For this review, take the finished solid that the model builds, in its own axes (mm). A direction names the side the tool comes from. Coordinates: 2 decimals unless noted, no trailing zeros. Write each loop counter-clockwise with the first axis right and the second up, starting at its lowest first coordinate (ties: lowest second). Pieces come first, ordered by that corner, then holes. Notation, with made-up numbers: (20, 15) - (75, 15) arc R28 cw to (75, 47) - close; hole circle Ø10 at (53.5, 50.5). An arc over 180 degrees is marked (long way). Write each question's results on one line, items separated by ' | '.
from build123d import *

# Parameters (mm, degrees)
CUT_EXTRUDE3_DEPTH           = 60
CUT_EXTRUDE5_DEPTH           = 2
CUT_EXTRUDE5_DEPTH_BACK      = 30
SKETCH9_R                    = 38
SKETCH9_R_2                  = 23
SKETCH19_W                   = 12
SKETCH19_H                   = 36.5
CUT_REVOLVE2_ANGLE           = 65
CUT_REVOLVE2_OTHER_WAY_ANGLE = 65
SKETCH21_W                   = 3.25
SKETCH21_H                   = 4
BOSS_EXTRUDE3_DEPTH          = 1.35
CIRPATTERN1_COUNT            = 5
CUT_EXTRUDE9_START           = -5
CUT_EXTRUDE9_DEPTH           = 5
SKETCH23_R                   = 10.5
CUT_EXTRUDE10_DEPTH          = 10
SKETCH24_W                   = 15
SKETCH24_H                   = 8
BOSS_EXTRUDE4_DEPTH          = 8
SKETCH26_W                   = 10
SKETCH26_H                   = 6
CUT_EXTRUDE11_DEPTH          = 10
SKETCH27_W                   = 4
SKETCH27_H                   = 5
CUT_EXTRUDE12_DEPTH          = 5
CUT_EXTRUDE14_DEPTH          = 2
CUT_EXTRUDE14_DEPTH_BACK     = 30
SKETCH29_R                   = 1
CUT_EXTRUDE15_DEPTH          = 15
FILLET1_R                    = 6
FILLET2_R                    = 8


# Read off the part's stored shape, not the designer's step: Cut-Extrude9
with BuildPart() as part:
    # Sketch1 → Revolve1 (revolve)
    with BuildSketch(Plane.XY, mode=Mode.PRIVATE) as revolve1_sk:
        with BuildLine():
            Line((0, 63.427876097), (32, 63.427876097))
            ThreePointArc((32, 63.427876097), (37.656854249, 61.084730346), (40, 55.427876097))
            Line((40, 55.427876097), (40, 28.846818009))
            ThreePointArc((40, 28.846818009), (38.792081772, 24.082439968), (35.460140376, 20.469057744))
            Line((35.460140376, 20.469057744), (28.539859624, 15.958818353))
            ThreePointArc((28.539859624, 15.958818353), (25.207918228, 12.345436129), (24, 7.581058088))
            Line((24, 7.581058088), (24, 3.25))
            Line((24, 3.25), (24.35, 3))
            Line((24.35, 3), (24.35, 0))
            Line((24.35, 0), (22.5, 0))
            Line((22.5, 0), (22.5, 12.5))
            ThreePointArc((22.5, 12.5), (22.353553391, 12.853553391), (22, 13))
            Line((22, 13), (0, 13))
            Line((0, 13), (0, 63.427876097))
        make_face()
    revolve(revolve1_sk.sketch.rotate(Axis((0, 0, 0), (0, 1, 0)), 90), axis=Axis((0, 0, 0), (0, 1, 0)))

    # Sketch11 → Cut-Extrude3 (cut)
    with BuildSketch(Plane(origin=(0, 13, 0), x_dir=(-1, 0, 0), z_dir=(0, -1, 0))):
        with BuildLine():
            Line((-21, 0), (21, 0))
            ThreePointArc((21, 0), (0, 21), (-21, 0))
        make_face()
    extrude(amount=-CUT_EXTRUDE3_DEPTH, mode=Mode.SUBTRACT)

    # Sketch9 → Cut-Extrude5 (cut, two sides: drawn at the far end of the back side and taken through both)
    with BuildSketch(Plane(origin=(0, 55.427876097, 0), x_dir=(1, 0, 0), z_dir=(0, 1, 0)).offset(-CUT_EXTRUDE5_DEPTH_BACK)):
        with Locations(Location((0, 0, 0), (0, 0, 270))):
            Circle(SKETCH9_R)
        with Locations(Location((0, 0, 0), (0, 0, 270))):
            Circle(SKETCH9_R_2, mode=Mode.SUBTRACT)
    extrude(amount=CUT_EXTRUDE5_DEPTH + CUT_EXTRUDE5_DEPTH_BACK, mode=Mode.SUBTRACT)

    # Sketch19 → Cut-Revolve2 (revolve, cut)
    with BuildSketch(Plane(origin=(0, 0, 0), x_dir=(0, 0, -1), z_dir=(1, 0, 0))):
        with Locations((-41.064715832, 37.177876097)):
            Rectangle(SKETCH19_W, SKETCH19_H)
    revolve(axis=Axis((0, 0, 0), (0, 1, 0)), revolution_arc=CUT_REVOLVE2_ANGLE, mode=Mode.SUBTRACT)

    # Sketch19 → Cut-Revolve2 other way (revolve, cut)
    with BuildSketch(Plane(origin=(0, 0, 0), x_dir=(0, 0, -1), z_dir=(1, 0, 0))):
        with Locations((-41.064715832, 37.177876097)):
            Rectangle(SKETCH19_W, SKETCH19_H)
    revolve(axis=Axis((0, 0, 0), (0, -1, 0)), revolution_arc=CUT_REVOLVE2_OTHER_WAY_ANGLE, mode=Mode.SUBTRACT)

    # Sketch21 → Boss-Extrude3 (add)
    with BuildSketch(Plane(origin=(0, 0, 22.5), x_dir=(-1, 0, 0), z_dir=(0, 0, -1))):
        with Locations((0, 2)):
            Rectangle(SKETCH21_W, SKETCH21_H)
    boss_extrude3 = extrude(amount=BOSS_EXTRUDE3_DEPTH)

    # CirPattern1: Boss-Extrude3 ×5 about axis
    cirpattern1_axis = Axis((0, 0, 0), (0, 1, 0))
    for i in range(1, CIRPATTERN1_COUNT):
        add(boss_extrude3.rotate(cirpattern1_axis, i * 360 / CIRPATTERN1_COUNT))

    # Cut-Extrude9 outline → Cut-Extrude9 (cut)
    with BuildSketch(Plane(origin=(0, 63.427876097, 0), x_dir=(1, 0, 0), z_dir=(0, 1, 0)).offset(CUT_EXTRUDE9_START)):
        with BuildLine():
            ThreePointArc((40, 0), (0, 40), (-40, 0))
            Line((-40, 0), (-21, 0))
            ThreePointArc((-21, 0), (0, 21), (21, 0))
            Line((21, 0), (40, 0))
        make_face()
    extrude(amount=CUT_EXTRUDE9_DEPTH, mode=Mode.SUBTRACT)

    # Sketch23 → Cut-Extrude10 (cut)
    with BuildSketch(Plane(origin=(0, 0, -40), x_dir=(-1, 0, 0), z_dir=(0, 0, -1))):
        with Locations((0, 42.137876097)):
            Circle(SKETCH23_R)
    extrude(amount=-CUT_EXTRUDE10_DEPTH, mode=Mode.SUBTRACT)

    # Sketch24 → Boss-Extrude4 (add)
    with BuildSketch(Plane(origin=(0, 58.427876097, 0), x_dir=(1, 0, 0), z_dir=(0, 1, 0))):
        with Locations((0, 30)):
            Rectangle(SKETCH24_W, SKETCH24_H)
    extrude(amount=-BOSS_EXTRUDE4_DEPTH)

    # Sketch26 → Cut-Extrude11 (cut)
    with BuildSketch(Plane(origin=(0, 58.427876097, 0), x_dir=(1, 0, 0), z_dir=(0, 1, 0))):
        with Locations((0, 30)):
            Rectangle(SKETCH26_W, SKETCH26_H)
    extrude(amount=-CUT_EXTRUDE11_DEPTH, mode=Mode.SUBTRACT)

    # Sketch27 → Cut-Extrude12 (cut)
    with BuildSketch(Plane(origin=(7.5, 0, 0), x_dir=(0, 0, -1), z_dir=(1, 0, 0))):
        with Locations((30, 53.927876097)):
            Rectangle(SKETCH27_W, SKETCH27_H)
    extrude(amount=-CUT_EXTRUDE12_DEPTH, mode=Mode.SUBTRACT)

    # Sketch28 → Cut-Extrude14 (cut, two sides: drawn at the far end of the back side and taken through both)
    with BuildSketch(Plane(origin=(0, 55.427876097, 0), x_dir=(1, 0, 0), z_dir=(0, 1, 0)).offset(-CUT_EXTRUDE14_DEPTH_BACK)):
        with BuildLine():
            Line((-22.912878475, -2), (22.912878475, -2))
            ThreePointArc((22.912878475, -2), (0, -23), (-22.912878475, -2))
        make_face()
    extrude(amount=CUT_EXTRUDE14_DEPTH + CUT_EXTRUDE14_DEPTH_BACK, mode=Mode.SUBTRACT)

    # Sketch29 → Cut-Extrude15 (cut)
    with BuildSketch(Plane(origin=(0, 0, 0), x_dir=(-1, 0, 0), z_dir=(0, 0, -1))):
        with Locations((-30.416198487, 60.927876097)):
            Circle(SKETCH29_R)
        with Locations((30.416198487, 60.927876097)):
            Circle(SKETCH29_R)
        with Locations((0, 60.927876097)):
            Circle(SKETCH29_R)
    extrude(amount=-CUT_EXTRUDE15_DEPTH, mode=Mode.SUBTRACT)

    # Fillet1
    fillet1_edges = [part.edges().sort_by_distance(p)[0] for p in [
        (21, 35.713938048, 0),
        (-21, 35.713938048, 0),
    ]]
    fillet(fillet1_edges, radius=FILLET1_R)

    # Fillet2
    fillet2_edges = [part.edges().sort_by_distance(p)[0] for p in [
        (-22.912878475, 41.427876097, 2),
        (22.912878475, 41.427876097, 2),
    ]]
    fillet(fillet2_edges, radius=FILLET2_R)


solid = part.part
Q1. For faces 1 (the face through (13, 4, -18)), 2 (the face through (-30.2, 59.95, 7.4)), 3 (the face through (20.122, 2.028, 6.514)), list the 3-axis set-ups (+Z, -Z, +X, -X, +Y, -Y) from which the entire face can be reached by the end or side of a thin tool; tool diameter is ignored.
Results found:
face 1: none | face 2: -Z | face 3: -Y
Q2. Take a section at C-C on y = 35. State the section outline as (x, z) points.
Results found:
outline: (-36.25, 16.9) arc R40 ccw to (-7.7, -39.25) - (-7.7, -37.21) arc R38 cw to (-34.44, 16.06) - close; (-21.08, -9.2) arc R23 ccw to (21.08, -9.2) arc R8 ccw to (13.75, 2) - (-13.75, 2) arc R8 ccw to start; (7.7, -39.25) arc R40 ccw to (36.25, 16.9) - (34.44, 16.06) arc R38 cw to (7.7, -37.21) - close; hole (-19.25, -8.4) arc R21 ccw to (19.25, -8.4) arc R6 ccw to (13.75, 0) - (-13.75, 0) arc R6 ccw to start
Q3. Take a section at A-A on y = 48. State the section outline as (x, z) points.
Results found:
outline: (-36.25, 16.9) arc R40 ccw to (-8.71, -39.04) - (-8.71, -36.99) arc R38 cw to (-34.44, 16.06) - close; (-21.08, -9.2) arc R23 ccw to (21.08, -9.2) arc R8 ccw to (13.75, 2) - (-13.75, 2) arc R8 ccw to start; (8.71, -39.04) arc R40 ccw to (36.25, 16.9) - (34.44, 16.06) arc R38 cw to (8.71, -36.99) - close; hole (-19.25, -8.4) arc R21 ccw to (19.25, -8.4) arc R6 ccw to (13.75, 0) - (-13.75, 0) arc R6 ccw to start
Q4. Mouldability with a two-part tool opening along X and no side actions: class faces 4 (the face through (25.62, 16.18, -13.32)), 5 (the face through (-12.45, 2.028, -17.097)) as pulls with the +X half, pulls with the -X half, needs draft (parallel to the pull), parting line crosses it, or undercut.
Results found:
face 4: parting line crosses it | face 5: undercut
Q5. For pin 1 (6.5 mm diameter, centred on x = -1, y = 54.5, fed in from +Z); pin 2 (1 mm diameter, centred on y = 19.5, z = -1.5, fed in from -X); pin 3 (0.6 mm diameter, centred on x = 30, y = 60.5, fed in from -Z); pin 4 (17 mm diameter, centred on x = 0, y = 42.14, fed in from +Z), all flat-tipped, find the tip position at first contact; note any pin that passes through.
Results found:
pin 1: z = 40 | pin 2: x = -34.71 | pin 3: z = 15 | pin 4: z = 2
Q6. Wall thickness on line 1 along Z through (x, y) = (8.5, 51.5); line 2 along X through (y, z) = (49.5, -12); line 3 along Y through (x, z) = (8, 15): over which ranges is each line inside the solid? List them lowest first. Write a range as from..to.
Results found:
line 1: -39.09..-37.04, -21.37..-19.2, 0..2 | line 2: -38.16..-36.06, -19.62..-17.23, 17.23..19.62, 36.06..38.16 | line 3: 13..25.43, 57.43..63.43
Q7. Take a section at B-B on y = 6. State the section outline as (x, z) points.
Results found:
outline: circle Ø48 at (0, 0); hole circle Ø45 at (0, 0)
